Part model, mm, in its own coordinate system. A direction names the side the tool comes from. Give positions to 0.01 mm unless a question says otherwise; leave off trailing zeros. Loops run counter-clockwise (first coordinate to the right, second up) from the corner with the lowest first, then second, coordinate; pieces in that order, holes last. Notation, with made-up numbers: M 1,39.25 L 27,39.25 A7 cw 27,51.25 Z; hole C -33,31.25 d3. An arc over 180 degrees is marked long. Answer in a Markdown table with one row per item.
from build123d import *

# Parameters (mm, degrees)
SKETCH1_W                = 48
SKETCH1_H                = 32
BOSS_EXTRUDE1_DEPTH      = 3
SKETCH2_W                = 48
SKETCH2_H                = 3
BOSS_EXTRUDE2_DEPTH      = 50
CUT_EXTRUDE1_DEPTH       = 67.400301204
CUT_EXTRUDE1_DEPTH_BACK  = 67.400301204
SKETCH3_R                = 2.5
F_5_0_5_DIAMETER_HOLE1_D = 5
KES_EKSTR_ZYON1_DEPTH    = 7


with BuildPart() as part:
    # Sketch1 → Boss-Extrude1 (new body)
    with BuildSketch(Plane(origin=(0, 0, 0), x_dir=(1, 0, 0), z_dir=(0, 1, 0))):
        Rectangle(SKETCH1_W, SKETCH1_H)
    extrude(amount=-BOSS_EXTRUDE1_DEPTH)

    # Sketch2 → Boss-Extrude2 (add)
    with BuildSketch(Plane.XZ.offset(3)):
        with Locations((0, 14.5)):
            Rectangle(SKETCH2_W, SKETCH2_H)
        with Locations((0, -14.5)):
            Rectangle(SKETCH2_W, SKETCH2_H)
    extrude(amount=BOSS_EXTRUDE2_DEPTH)

    # Sketch3 → Cut-Extrude1 (cut, two sides: drawn at the far end of the back side and taken through both)
    with BuildSketch(Plane.XY.offset(16).offset(-CUT_EXTRUDE1_DEPTH_BACK)):
        with BuildLine():
            Line((24, -53), (24, -10.287171893))
            Line((24, -10.287171893), (6.367730582, -48.907233604))
            ThreePointArc((6.367730582, -48.907233604), (3.784796178, -51.8885752), (-8.6e-08, -53))
            Line((-8.6e-08, -53), (24, -53))
        make_face()
        with BuildLine():
            Line((-24, -53), (-8.6e-08, -53))
            ThreePointArc((-8.6e-08, -53), (-3.784796251, -51.888575154), (-6.367730582, -48.907233604))
            Line((-6.367730582, -48.907233604), (-24, -10.287171893))
            Line((-24, -10.287171893), (-24, -53))
        make_face()
        with Locations((0, -46)):
            Circle(SKETCH3_R)
    extrude(amount=CUT_EXTRUDE1_DEPTH + CUT_EXTRUDE1_DEPTH_BACK, mode=Mode.SUBTRACT)

    # Ø5.0 (5) Diameter Hole1 (through all)
    with Locations(Plane(origin=(0, 0, 0), x_dir=(1, 0, 0), z_dir=(0, 1, 0))):
        with Locations((-15, -9), (-15, 9), (15, 9), (15, -9)):
            Hole(F_5_0_5_DIAMETER_HOLE1_D / 2)

    # Çizim1 → Kes-Ekstrüzyon1 (cut)
    with BuildSketch(Plane(origin=(0, 0, 0), x_dir=(1, 0, 0), z_dir=(0, 1, 0))):
        with BuildLine():
            Line((-4, 1), (-4, -1))
            ThreePointArc((-4, -1), (0, -5), (4, -1))
            Line((4, -1), (4, 1))
            ThreePointArc((4, 1), (0, 5), (-4, 1))
        make_face()
    extrude(amount=-KES_EKSTR_ZYON1_DEPTH, mode=Mode.SUBTRACT)


solid = part.part
(1) Saw through at C-C (x = -15). Write the cut outline in (y, z), plus the area to 3 significant figures.
Recorded:
| item | result |
|---|---|
| outline | M -30,-16 L 0,-16 L 0,-11.5 L -3,-11.5 L -3,-13 L -30,-13 Z; M -30,13 L -3,13 L -3,11.5 L 0,11.5 L 0,16 L -30,16 Z; M -3,-6.5 L 0,-6.5 L 0,6.5 L -3,6.5 Z |
| area | 228 mm^2 |
(2) Saw through at B-B (y = -46). Write the cut outline in (x, z).
Recorded:
| item | result |
|---|---|
| outline | M -7.7,-16 L -2.5,-16 L -2.5,-13 L -7.7,-13 Z; M -7.7,13 L -2.5,13 L -2.5,16 L -7.7,16 Z; M 2.5,-16 L 7.7,-16 L 7.7,-13 L 2.5,-13 Z; M 2.5,13 L 7.7,13 L 7.7,16 L 2.5,16 Z |
(3) Saw through at A-A (z = 9). Write the cut outline in (x, y).
Recorded:
| item | result |
|---|---|
| outline | M -24,-3 L -17.5,-3 L -17.5,0 L -24,0 Z; M -12.5,-3 L 12.5,-3 L 12.5,0 L -12.5,0 Z; M 17.5,-3 L 24,-3 L 24,0 L 17.5,0 Z |
(4) Which spindle directions (+Z, -Z, +X, -X, +Y, -Y) get a long thin tool onto all of the face, cutting with end or side? Do faces 5 (the face through (-24, -2.8, -0.2)), 6 (the face through (0, -22, -13)), 7 (the face through (4, -1, 0)). Say none if no direction does.
Recorded:
| item | result |
|---|---|
| face 5 | +Z, -Z, -X, +Y, -Y |
| face 6 | +X, -X, -Y |
| face 7 | +Y, -Y |
(5) Drill centre lines: line 1 along Z through (x, y) = (-15, -1.15); line 2 along Z through (x, y) = (-21, -7); line 3 along Y through (x, z) = (19, 5.5). Where is each one in solid material? Low to high.
Recorded:
| item | result |
|---|---|
| line 1 | z = -16 to -11.5, -6.5 to 6.5, 11.5 to 16 |
| line 2 | z = -16 to -13, 13 to 16 |
| line 3 | y = -3 to 0 |
(6) Saw through at D-D (x = -1.5). Write the cut outline in (y, z), plus the area to 3 significant figures.
Recorded:
| item | result |
|---|---|
| outline | M -52.84,-16 L -48,-16 L -48,-13 L -52.84,-13 Z; M -52.84,13 L -48,13 L -48,16 L -52.84,16 Z; M -44,-16 L 0,-16 L 0,-4.71 L -3,-4.71 L -3,-13 L -44,-13 Z; M -44,13 L -3,13 L -3,4.71 L 0,4.71 L 0,16 L -44,16 Z |
| area | 343 mm^2 |
(7) Pin check, flat tip, straight feed: pin 1 Ø6 at (x, z) = (-13.5, -3.5) entering from -Y. Stop position of the tip, or through.
Recorded:
| item | result |
|---|---|
| pin 1 | stops at y = -3 |
(8) Pull direction Y, two halves, no side cores. Call faces 1 (the face through (-0.54, -48.44, -14.52)), 2 (the face through (-13, -1.5, -7.5)), 3 (the face through (5, 0, 0)), 4 (the face through (15.307, -29.327, -14.521)): +Y half, -Y half, draft (parallel to the pull), parting line (faces both ways), or undercut.
Recorded:
| item | result |
|---|---|
| face 1 | undercut |
| face 2 | draft |
| face 3 | +Y half |
| face 4 | -Y half |
